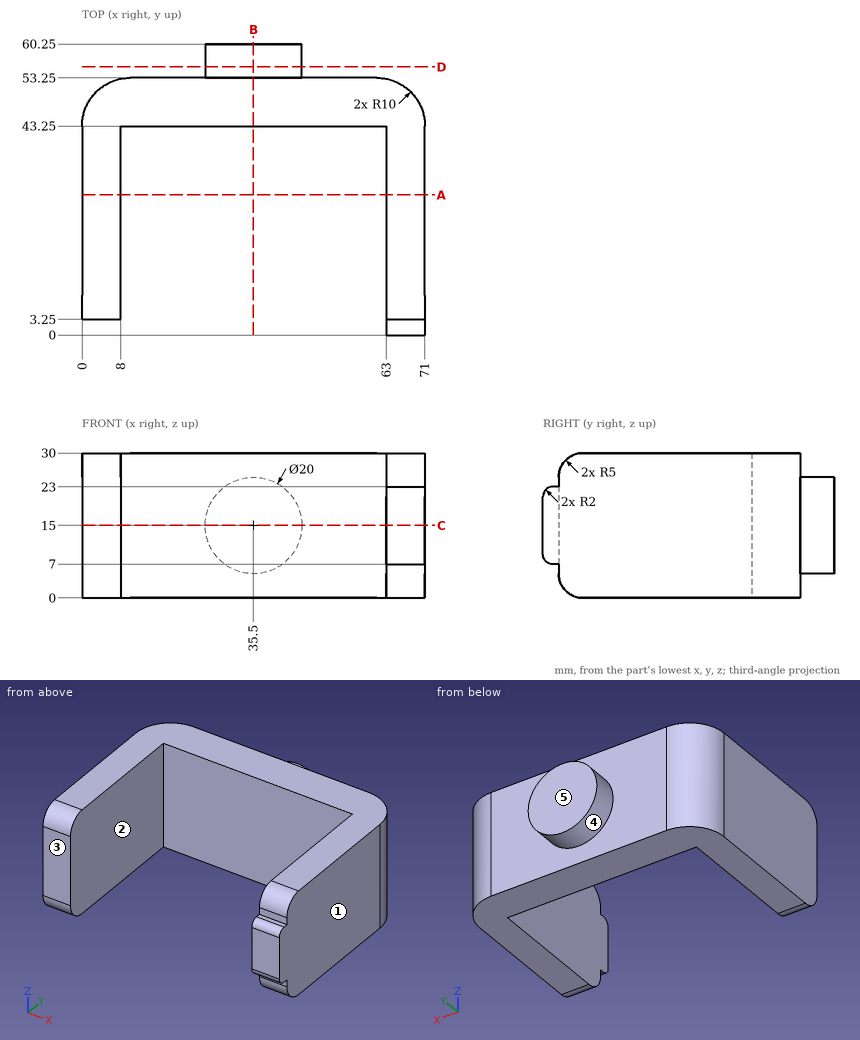
Answer from the drawing. Dimensions are ordinates in mm from the lowest x, y and z of the part. A direction names the side the tool comes from. Round coordinates to 2 decimals unless told otherwise and drop trailing zeros. Loops run counter-clockwise (first coordinate to the right, second up) from the corner with the lowest first, then second, coordinate; pieces in that order, holes last.
Q1. Section A-A on y = 29 is taken. Write down the section's boundary in (x, z), and give its area (3 significant figures).
Q2. Section B-B on x = 35.5 is taken. Write down the section's boundary in (y, z), and give its area (3 significant figures).
Q3. Section C-C on z = 15 is taken. Write down the section's boundary in (x, y).
Q4. Which of the six approach directions +Z, -Z, +X, -X, +Y, -Y give full straight-line access (tool end or side, diameter ignored) to the marked faces 1, 2, 3, 4 and 5?
Q5. Consider probe 1 along X at (y, z) = (13.5, 5.25); probe 2 along Y at (x, z) = (19, 13.5); probe 3 along Y at (x, z) = (27.5, 10.75). Determine where each line is inside the solid, lowest interval first.
Q6. Each of these flat-tipped pins is pushed along its axis until it touches: pin 1 (2.5 mm diameter, centred on x = 2, z = 10, fed in from -Y); pin 2 (0.6 mm diameter, centred on x = 69, y = 2.5, fed in from +Z); pin 3 (1 mm diameter, centred on x = 38, z = 7.5, fed in from -Y); pin 4 (1.5 mm diameter, centred on x = 50, y = 41.5, fed in from +Z). Where does it stop, or does it pass through?
Q7. Section D-D on y = 55.5 is taken. Write down the section's boundary in (x, z).
Output:
1. outline: (0, 0) - (8, 0) - (8, 30) - (0, 30) - close; (63, 0) - (71, 0) - (71, 30) - (63, 30) - close
1. area: 480 mm2
2. outline: (43.25, 0) - (53.25, 0) - (53.25, 5) - (60.25, 5) - (60.25, 25) - (53.25, 25) - (53.25, 30) - (43.25, 30) - close
2. area: 440 mm2
3. outline: (0, 3.25) - (8, 3.25) - (8, 43.25) - (63, 43.25) - (63, 0) - (71, 0) - (71, 43.25) arc R10 ccw to (61, 53.25) - (45.5, 53.25) - (45.5, 60.25) - (25.5, 60.25) - (25.5, 53.25) - (10, 53.25) arc R10 ccw to (0, 43.25) - close
4. face 1: +Z, -Z, +X, +Y, -Y
4. face 2: +Z, -Z, -Y
4. face 3: +Z, -Z, -X, -Y
4. face 4: +Y
4. face 5: +Z, -Z, +X, -X, +Y
5. probe 1: x = 0 to 8, 63 to 71
5. probe 2: y = 43.25 to 53.25
5. probe 3: y = 43.25 to 60.25
6. pin 1: stops at y = 3.25
6. pin 2: stops at z = 23
6. pin 3: stops at y = 43.25
6. pin 4: passes through
7. outline: circle Ø20 at (35.5, 15)
